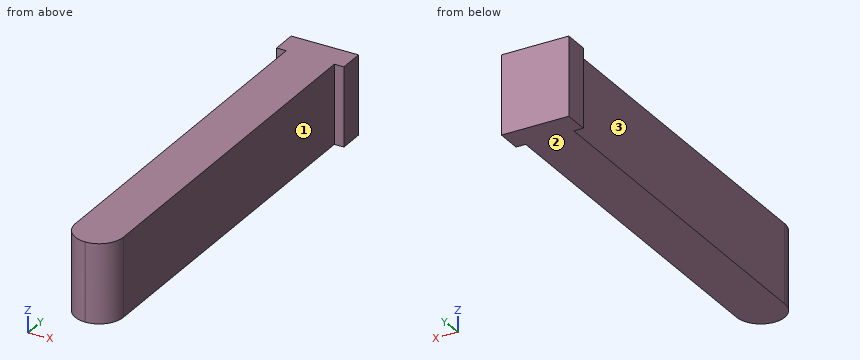
Autodesk Fusion 360 part; units mm, degrees
sketch "Sketch1" plane through (0, 0, 0) normal (0, 0, 1) x (1, 0, 0)
  line L0 (0, 0) -> (-1.75, 0)
  line L1 (-1.75, 0) -> (-1.75, -1.3)
  line L2 (-1.75, -1.3) -> (-1.25, -1.3)
  line L3 (-1.25, -1.3) -> (-1.25, -21.3)
  line L4 (-1.25, -21.3) -> (1.25, -21.3)
  line L5 (1.25, -21.3) -> (1.25, -1.3)
  line L6 (1.25, -1.3) -> (1.75, -1.3)
  line L7 (1.75, -1.3) -> (1.75, 0)
  line L8 (1.75, 0) -> (0, 0)
  line L9 (1.25, -1.3) -> (-1.25, -1.3) construction
  dimension "d1" = 3.5
  dimension "d2" = 1.3
  dimension "d3" = 20
  dimension "d4" = 2.5
extrude "Extrude1" add sketch "Sketch1" along normal blind 4.1
fillet "Fillet1" radius 1.25 2 edges at (1.25, -21.3, 2.05) (-1.25, -21.3, 2.05)
Geometry check sheet. Reference: the model listing, model coordinates, mm. Face numbers are marked on the shaded views. A direction names the side the tool comes from. Give positions to 0.01 mm unless a question says otherwise; leave off trailing zeros. Order: outer loops, then holes, each group sorted by start corner. A loop starts at its lowest first (then second) coordinate and runs counter-clockwise, first axis right, second up. Notation, with made-up numbers: (87, -16.5) - (127, -16.5) arc R16 cw to (127, -0.5) - close; hole circle Ø2 at (42, -37.5). An arc over 180 degrees is marked (long way). Answer as a JSON object with one key per item and string values.
(1) Cross-section at B-B (x = -1.5). Record the cut outline in (y, z), then the cut area to 3 significant figures.
Report:
{"outline": "(-1.3, 0) - (0, 0) - (0, 4.1) - (-1.3, 4.1) - close", "area": "5.33 mm^2"}
(2) Depth check by flat-ended pin: pin 1 Ø2 at (y, z) = (-9.5, 1.5) entering from +X. Enter the tip coordinate at first touch or a pass-through.
Report:
{"pin 1": "x = 1.25"}
(3) Cross-section at C-C (y = -11.5). Record the cut outline in (x, z).
Report:
{"outline": "(-1.25, 0) - (1.25, 0) - (1.25, 4.1) - (-1.25, 4.1) - close"}
(4) Tool access check on the marked faces 1, 2 and 3. Record the directions out of +Z, -Z, +X, -X, +Y, -Y that give a thin tool (end or side, any length) a straight path to the whole face; none if there is none.
Report:
{"face 1": "+Z, -Z, +X, -Y", "face 2": "-Z, +X, -X, +Y, -Y", "face 3": "+Z, -Z, -X, -Y"}
(5) Material ranges on line 1 (X direction, y = -7.5, z = 3.1); line 2 (Y direction, x = -1.3, z = 0.5); line 3 (Y direction, x = -0.6, z = 3.5), recorded low to high.
Report:
{"line 1": "-1.25 to 1.25", "line 2": "-1.3 to 0", "line 3": "-21.15 to 0"}
